from build123d import *

# Parameters (mm, degrees)
SKETCH1_W           = 50
SKETCH1_H           = 50
BOSS_EXTRUDE1_DEPTH = 10
BOSS_EXTRUDE2_DEPTH = 10
BOSS_EXTRUDE3_START = -10
BOSS_EXTRUDE3_DEPTH = 10
SKETCH4_R           = 12
CUT_EXTRUDE2_DEPTH  = 120


with BuildPart() as part:
    # Sketch1 → Boss-Extrude1 (new body)
    with BuildSketch(Plane.XY):
        with Locations((25, 25)):
            Rectangle(SKETCH1_W, SKETCH1_H)
    extrude(amount=BOSS_EXTRUDE1_DEPTH)

    # Sketch2 → Boss-Extrude2 (add)
    with BuildSketch(Plane(origin=(0, 0, 0), x_dir=(1, 0, 0), z_dir=(0, 1, 0))):
        with BuildLine():
            Line((0, 0), (49.911002168, 0))
            Line((49.911002168, 0), (49.911002168, 30))
            ThreePointArc((49.911002168, 30), (44.053137792, 44.142135624), (29.911002168, 50))
            Line((29.911002168, 50), (20, 50))
            ThreePointArc((20, 50), (5.857864376, 44.142135624), (0, 30))
            Line((0, 30), (0, 0))
        make_face()
    extrude(amount=BOSS_EXTRUDE2_DEPTH)

    # Sketch3 → Boss-Extrude3 (add)
    with BuildSketch(Plane(origin=(0, 50, 0), x_dir=(1, 0, 0), z_dir=(0, 1, 0)).offset(BOSS_EXTRUDE3_START)):
        with BuildLine():
            Line((0, 0), (49.911002168, 0))
            Line((49.911002168, 0), (49.911002168, 30))
            ThreePointArc((49.911002168, 30), (44.053137792, 44.142135624), (29.911002168, 50))
            Line((29.911002168, 50), (20, 50))
            ThreePointArc((20, 50), (5.857864376, 44.142135624), (0, 30))
            Line((0, 30), (0, 0))
        make_face()
    extrude(amount=BOSS_EXTRUDE3_DEPTH)

    # Sketch4 → Cut-Extrude2 (cut)
    with BuildSketch(Plane(origin=(0, 50, 0), x_dir=(1, 0, 0), z_dir=(0, 1, 0))):
        with Locations(Location((24.659042371, 30, 0), (0, 0, 270))):
            Circle(SKETCH4_R)
    extrude(amount=-CUT_EXTRUDE2_DEPTH, mode=Mode.SUBTRACT)


solid = part.part
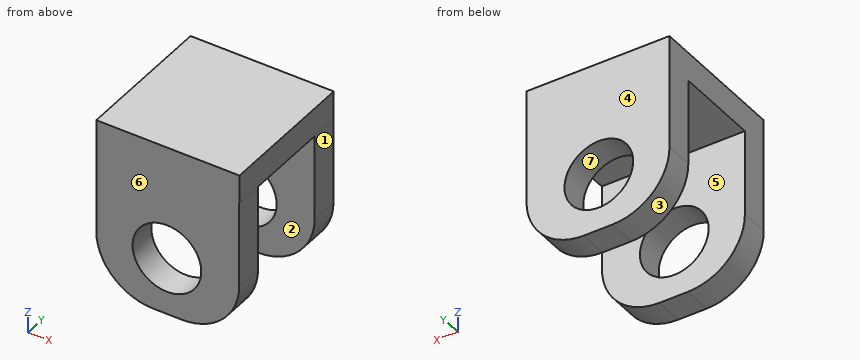
The model under review builds one solid part; all positions refer to its coordinate system, in mm. Face numbers are marked on the shaded views. A direction names the side the tool comes from. Coordinates: 2 decimals unless noted, no trailing zeros. Loops run counter-clockwise (first coordinate to the right, second up) from the corner with the lowest first, then second, coordinate; pieces in that order, holes last.
(1) Draft analysis for pull direction Y (two halves, no side actions). For the marked faces 4, 5, 6 and 7, state which applies: +Y half, -Y half, draft (parallel to the pull), parting line (faces both ways), or undercut.
Determined:
face 4: +Y half
face 5: undercut
face 6: -Y half
face 7: draft
(2) Wall thickness on L1, parallel to X at y = 45, z = -30; L2, parallel to Y at x = 15, z = -45.5; L3, parallel to Z at x = 11.5, y = 26: over which ranges is each line inside the solid? List them lowest first.
Determined:
L1: x = 0 to 12.66, 36.66 to 49.91
L2: y = 0 to 10, 40 to 50
L3: z = 0 to 10
(3) Consider section B-B, the plane x = 8. Give the boundary of the cut face in (y, z), plus the area to 3 significant figures.
Determined:
outline: (0, -46) - (10, -46) - (10, 0) - (40, 0) - (40, -46) - (50, -46) - (50, 10) - (0, 10) - close
area: 1,420 mm2
(4) Consider section D-D, the plane x = 27.5. Give the boundary of the cut face in (y, z), plus the area to 3 significant figures.
Determined:
outline: (0, -50) - (10, -50) - (10, -41.66) - (0, -41.66) - close; (0, -18.34) - (10, -18.34) - (10, 0) - (40, 0) - (40, -18.34) - (50, -18.34) - (50, 10) - (0, 10) - close; (40, -50) - (50, -50) - (50, -41.66) - (40, -41.66) - close
area: 1,030 mm2
(5) Tool access review of the marked faces 1, 2 and 3: name each direction out of +Z, -Z, +X, -X, +Y, -Y from which nothing blocks a thin tool from reaching the whole face with its end or side.
Determined:
face 1: -Z, +X, +Y, -Y
face 2: -Z, +X, -X
face 3: -Z, -X, +Y, -Y
(6) Consider section C-C, the plane z = -32. Give the boundary of the cut face in (x, y), plus the area to 3 significant figures.
Determined:
outline: (0.1, 0) - (12.83, 0) - (12.83, 10) - (0.1, 10) - close; (0.1, 40) - (12.83, 40) - (12.83, 50) - (0.1, 50) - close; (36.49, 0) - (49.81, 0) - (49.81, 10) - (36.49, 10) - close; (36.49, 40) - (49.81, 40) - (49.81, 50) - (36.49, 50) - close
area: 521 mm2
(7) Consider section A-A, the plane z = -15. Give the boundary of the cut face in (x, y), plus the area to 3 significant figures.
Determined:
outline: (0, 0) - (49.91, 0) - (49.91, 10) - (0, 10) - close; (0, 40) - (49.91, 40) - (49.91, 50) - (0, 50) - close
area: 998 mm2
(8) Insertion check: P1, Ø1, axis at x = 13, z = -22.5, coming from the -Y side; P2, Ø5, axis at y = 4.5, z = -14.5, coming from the +X side; P3, Ø19, axis at x = 24.66, z = -30, coming from the -Y side; P4, Ø4, axis at x = 21.5, y = 26, coming from the -Z side. Each pin has a flat end and moves straight along its axis. Give the tip position at first contact, or say it passes through.
Determined:
P1: stops at y = 0
P2: stops at x = 49.91
P3: passes through
P4: stops at z = 0
